from build123d import *

# Parameters (mm, degrees)
SKETCH1_W           = 30
SKETCH1_H           = 50
BOSS_EXTRUDE1_DEPTH = 3
BOSS_EXTRUDE2_DEPTH = 30
FILLET1_R           = 3
FILLET2_R           = 1


with BuildPart() as part:
    # Sketch1 → Boss-Extrude1 (new body)
    with BuildSketch(Plane.XY):
        with Locations((15, 25)):
            Rectangle(SKETCH1_W, SKETCH1_H)
    extrude(amount=BOSS_EXTRUDE1_DEPTH)

    # Sketch2 → Boss-Extrude2 (add)
    with BuildSketch(Plane.XY.offset(3)):
        Polygon((0, 50), (30, 50), (30, 0), (27, 0), (27, 47), (0, 47), align=None)
        Polygon((0, 40.9), (20.9, 40.9), (20.9, 0), (17.9, 0), (17.9, 37.9), (0, 37.9), align=None)
    extrude(amount=BOSS_EXTRUDE2_DEPTH)

    # Fillet1
    fillet1_edges = [part.edges().sort_by_distance(p)[0] for p in [
        (13.5, 47, 3),
        (27, 23.5, 3),
        (8.95, 37.9, 3),
        (17.9, 18.95, 3),
        (17.9, 37.9, 18),
        (20.9, 20.45, 3),
        (10.45, 40.9, 3),
    ]]
    fillet(fillet1_edges, radius=FILLET1_R)

    # Fillet2
    fillet2_edges = [part.edges().sort_by_distance(p)[0] for p in [
        (13.5, 47, 33),
        (27, 23.5, 33),
        (20.9, 20.45, 33),
        (10.45, 40.9, 33),
    ]]
    fillet(fillet2_edges, radius=FILLET2_R)


solid = part.part
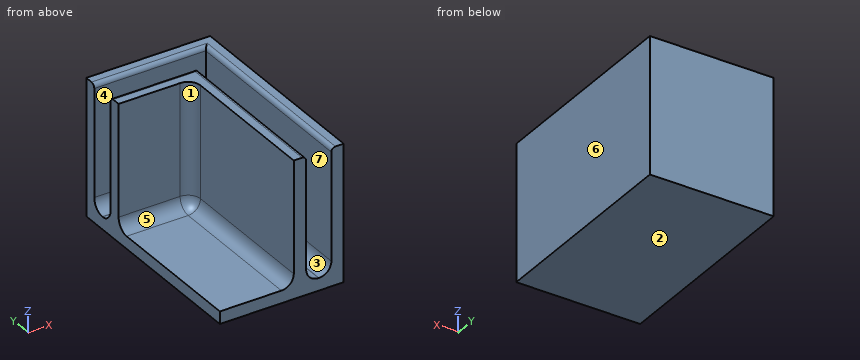
Check sheet for the modelled part. Datum: model origin and axes. Units: mm. Face numbers are marked on the shaded views. A direction names the side the tool comes from. Round coordinates to 2 decimals unless told otherwise and drop trailing zeros. Loops run counter-clockwise (first coordinate to the right, second up) from the corner with the lowest first, then second, coordinate; pieces in that order, holes last.
1. Sectioned sample at B-B on y = 9. Record the boundary of the cut face in (x, z).
2. Sectioned sample at D-D on x = 18.75. Record the boundary of the cut face in (y, z).
3. Set-up check for the marked faces 1, 2, 3 and 4: record each of +Z, -Z, +X, -X, +Y, -Y from which the full face is reachable in a straight line by a thin tool's end or side.
4. Mould release check, pull along X, two halves, no side actions. Record for the marked faces 5, 6 and 7: released by +X, released by -X, zero draft, split by the parting line, or undercut.
5. Scan lines: probe 1 along X at (y, z) = (11, 10); probe 2 along Y at (x, z) = (19.75, 13); probe 3 along Y at (x, z) = (4.25, 23.5). Record each from-to range of solid material in increasing order.
6. Sectioned sample at A-A on z = 24.5. Record the boundary of the cut face in (x, y), and give its area (3 significant figures).
7. Sectioned sample at C-C on x = 4.5. Record the boundary of the cut face in (y, z), and give its area (3 significant figures).
8. Gauge pin test, flat ends, axial feed: pin 1 Ø1.5 at (x, y) = (23, 31.5) entering from +Z; pin 2 Ø7.5 at (x, y) = (11, 13.5) entering from +Z; pin 3 Ø16.5 at (x, z) = (8, 20.5) entering from -Y. Record the tip position at first contact, or that the pin passes through.
Recorded:
1. outline: (0, 0) - (30, 0) - (30, 33) - (28, 33) arc R1 ccw to (27, 32) - (27, 6) arc R3 cw to (24, 3) - (23.9, 3) arc R3 cw to (20.9, 6) - (20.9, 32) arc R1 ccw to (19.9, 33) - (17.9, 33) - (17.9, 6) arc R3 cw to (14.9, 3) - (0, 3) - close
2. outline: (0, 0) - (50, 0) - (50, 33) - (48, 33) arc R1 ccw to (47, 32) - (47, 6) arc R3 cw to (44, 3) - (43.9, 3) arc R3 cw to (40.9, 6) - (40.9, 32) arc R1 ccw to (39.9, 33) - (0, 33) - close
3. face 1: +Z, -X, -Y
3. face 2: -Z, +X, -X, +Y, -Y
3. face 3: +Z, -Y
3. face 4: +Z, -X
4. face 5: zero draft
4. face 6: released by +X
4. face 7: undercut
5. probe 1: x = 17.9 to 20.9, 27 to 30
5. probe 2: y = 0 to 40.9, 47 to 50
5. probe 3: y = 37.9 to 40.9, 47 to 50
6. outline: (0, 37.9) - (14.9, 37.9) arc R3 cw to (17.9, 34.9) - (17.9, 0) - (20.9, 0) - (20.9, 40.9) - (0, 40.9) - close; (0, 47) - (27, 47) - (27, 0) - (30, 0) - (30, 50) - (0, 50) - close
6. area: 409 mm2
7. outline: (0, 0) - (50, 0) - (50, 33) - (48, 33) arc R1 ccw to (47, 32) - (47, 6) arc R3 cw to (44, 3) - (43.9, 3) arc R3 cw to (40.9, 6) - (40.9, 32) arc R1 ccw to (39.9, 33) - (37.9, 33) - (37.9, 6) arc R3 cw to (34.9, 3) - (0, 3) - close
7. area: 335 mm2
8. pin 1: stops at z = 3.49
8. pin 2: stops at z = 3
8. pin 3: stops at y = 37.58
